Autodesk Fusion 360 part; units mm, degrees
sketch "Esquisse1" plane through (0, 0, 0) normal (0, 0, 1) x (1, 0, 0)
  line L0 (-50, 50.0735) -> (20, 50.0735)
  line L1 (20, 50.0735) -> (20, 34.0735)
  line L2 (20, 34.0735) -> (-50, 34.0735)
  line L3 (-50, 34.0735) -> (-50, 50.0735)
  circle A0 centre (-40, 42) radius 1.65
  circle A1 centre (10, 42) radius 1.65
  line L4 (7.25, 40.4123) -> (10, 38.8246)
  line L5 (10, 38.8246) -> (12.75, 40.4123)
  line L6 (12.75, 40.4123) -> (12.75, 43.5877)
  line L7 (12.75, 43.5877) -> (10, 45.1754)
  line L8 (10, 45.1754) -> (7.25, 43.5877)
  line L9 (7.25, 43.5877) -> (7.25, 40.4123)
  line L10 (-42.75, 40.4123) -> (-40, 38.8246)
  line L11 (-40, 38.8246) -> (-37.25, 40.4123)
  line L12 (-37.25, 40.4123) -> (-37.25, 43.5877)
  line L13 (-37.25, 43.5877) -> (-40, 45.1754)
  line L14 (-40, 45.1754) -> (-42.75, 43.5877)
  line L15 (-42.75, 43.5877) -> (-42.75, 40.4123)
  point P0 (10, 42)
  point P1 (-40, 42)
  dimension "d2" = 16
  dimension "d3" = 70
  dimension "d5" = 3.3
  dimension "d6" = 3.3
  dimension "d7" = 10
  dimension "d8" = 10
  dimension "d23" = 2.75
  dimension "d24" = 2.75
  dimension "d37" = 50
extrude "Extrusion1" add sketch "Esquisse1" along normal blind 20 contours L0 L1 L2 L3 | A0 | A1 | L4 L5 L6 L7 L8 L9 | L10 L11 L12 L13 L14 L15
extrude "Extrusion7" cut sketch "Esquisse1" along normal blind 19 and the other way blind 0 contours A0 | A1
extrude "Extrusion6" cut sketch "Esquisse1" along normal blind 13 and the other way blind -11 contours L4 L5 L6 L7 L8 L9 | L10 L11 L12 L13 L14 L15
sketch "Esquisse2" plane through (0, 0, 0) normal (0, 0, 1) x (1, 0, 0)
  line L0 (-26.6171, 50.3546) -> (-3.6171, 50.3546)
  line L1 (-3.6171, 50.3546) -> (-3.6171, 33.8546)
  line L2 (-3.6171, 33.8546) -> (-26.6171, 33.8546)
  line L3 (-26.6171, 33.8546) -> (-26.6171, 50.3546)
  dimension "d11" = 23
  dimension "d12" = 16.5
extrude "Extrusion2" cut sketch "Esquisse2" along normal blind 12.7
sketch "Esquisse3" plane through (0, 0, 0) normal (0, 1, 0) x (1, 0, 0)
  circle A0 centre (-28.6171, -7) radius 1
  circle A1 centre (-1.6171, -7) radius 1
  line L0 (-26.6171, 0) -> (-26.6171, -12.7)
  line L1 (-3.6171, -12.7) -> (-3.6171, 0)
  dimension "d15" = 2
  dimension "d16" = 2
  dimension "d17" = 2
  dimension "d18" = 2
extrude "Extrusion3" cut sketch "Esquisse3" along normal blind 51 and the other way blind -34
extrude "Extrusion4" cut sketch "Esquisse1" along normal blind 8 and the other way blind -5 contours L10 L11 L12 L13 L14 L15
extrude "Extrusion5" cut sketch "Esquisse1" along normal blind 8 and the other way blind -5 contours L4 L5 L6 L7 L8 L9
equation "d6 = d5"
equation "d16 = d15"
Input: part model. Units: mm. Frame: model coordinates. A direction names the side the tool comes from. Coordinates: 2 decimals unless noted, no trailing zeros. Write each loop counter-clockwise with the first axis right and the second up, starting at its lowest first coordinate (ties: lowest second). Pieces come first, ordered by that corner, then holes. Notation, with made-up numbers: (21, 61) -> (51, 61) arc R31 cw to (51, 98) -> close; hole circle Ø1 at (-30, 41). An arc over 180 degrees is marked (long way). Write each question's results on one line, items separated by ' | '.
Item 1: Section query D-D on z = 4.25. Return loops of the section in (x, y), plus the area to 3 significant figures.
Conclusion:
outline: (-50, 34.07) -> (-26.62, 34.07) -> (-26.62, 50.07) -> (-50, 50.07) -> close; (-3.62, 34.07) -> (20, 34.07) -> (20, 50.07) -> (-3.62, 50.07) -> close; hole circle Ø3.3 at (-40, 42); hole circle Ø3.3 at (10, 42) | area: 735 mm^2
Item 2: Section query B-B on z = 7. Return loops of the section in (x, y), plus the area to 3 significant figures.
Conclusion:
outline: (-50, 34.07) -> (-29.62, 34.07) -> (-29.62, 50.07) -> (-50, 50.07) -> close; (-27.62, 34.07) -> (-26.62, 34.07) -> (-26.62, 50.07) -> (-27.62, 50.07) -> close; (-3.62, 34.07) -> (-2.62, 34.07) -> (-2.62, 50.07) -> (-3.62, 50.07) -> close; (-0.62, 34.07) -> (20, 34.07) -> (20, 50.07) -> (-0.62, 50.07) -> close; hole (-42.75, 40.41) -> (-40, 38.82) -> (-37.25, 40.41) -> (-37.25, 43.59) -> (-40, 45.18) -> (-42.75, 43.59) -> close; hole (7.25, 40.41) -> (10, 38.82) -> (12.75, 40.41) -> (12.75, 43.59) -> (10, 45.18) -> (7.25, 43.59) -> close | area: 636 mm^2
Item 3: Material intervals for probe 1 along Z at (x, y) = (9, 39.5); probe 2 along X at (y, z) = (35.5, 11.75); probe 3 along Y at (x, z) = (10, 16.1), sorted ascending.
Conclusion:
probe 1: z = 0 to 5, 8 to 11, 13 to 20 | probe 2: x = -50 to -26.62, -3.62 to 20 | probe 3: y = 34.07 to 40.35, 43.65 to 50.07
Item 4: Pin query (flat end, axial travel): pin 1 Ø5.5 at (x, y) = (10, 42) entering from -Z; pin 2 Ø5 at (x, y) = (-16.5, 43) entering from -Z. Return the tip coordinate at first contact, or that it passes through.
Conclusion:
pin 1: stops at z = 0 | pin 2: stops at z = 12.7
Item 5: Mould query, pull axis X, two halves, no side actions, for faces 4 (the flat face through (8.64, 44.39, 6.48)), 5 (the flat face through (-38, 44, 0)), 6 (the flat face through (20, 42, 10)). Classes: +X half, -X half, draft (parallel to the pull), parting line (faces both ways), or undercut.
Conclusion:
face 4: undercut | face 5: draft | face 6: +X half
Item 6: Section query C-C on y = 47.5. Return loops of the section in (x, z), plus the area to 3 significant figures.
Conclusion:
outline: (-50, 0) -> (-26.62, 0) -> (-26.62, 12.7) -> (-3.62, 12.7) -> (-3.62, 0) -> (20, 0) -> (20, 20) -> (-50, 20) -> close; hole circle Ø2 at (-28.62, 7); hole circle Ø2 at (-1.62, 7) | area: 1,100 mm^2
Item 7: Set-up query: faces 1 (the flat face through (-41.394, 39.63, 6.479)), 2 (the flat face through (-15, 34.074, 14)), 3 (the cylindrical face through (10.89, 40.61, 9.48)). Return all of +Z, -Z, +X, -X, +Y, -Y with unobstructed straight access to the full face (end or side cutting, diameter ignored); none if empty.
Conclusion:
face 1: none | face 2: +Z, -Z, +X, -X, -Y | face 3: -Z
Item 8: Section query A-A on z = 12. Return loops of the section in (x, y).
Conclusion:
outline: (-50, 34.07) -> (-26.62, 34.07) -> (-26.62, 50.07) -> (-50, 50.07) -> close; (-3.62, 34.07) -> (20, 34.07) -> (20, 50.07) -> (-3.62, 50.07) -> close; hole (-42.75, 40.41) -> (-40, 38.82) -> (-37.25, 40.41) -> (-37.25, 43.59) -> (-40, 45.18) -> (-42.75, 43.59) -> close; hole (7.25, 40.41) -> (10, 38.82) -> (12.75, 40.41) -> (12.75, 43.59) -> (10, 45.18) -> (7.25, 43.59) -> close
